Work out the finished part from the listing and answer in its coordinate system (mm). Give positions to 0.01 mm unless a question says otherwise; leave off trailing zeros. Write each loop counter-clockwise with the first axis right and the second up, starting at its lowest first coordinate (ties: lowest second). Pieces come first, ordered by that corner, then holes. Notation, with made-up numbers: (5.25, -28.5) - (24.25, -28.5) arc R12 cw to (24.25, -7.5) - close; hole circle Ø8 at (64.25, -7). An arc over 180 degrees is marked (long way). Write each question's results on one line, items separated by ' | '. Start each with the question number.
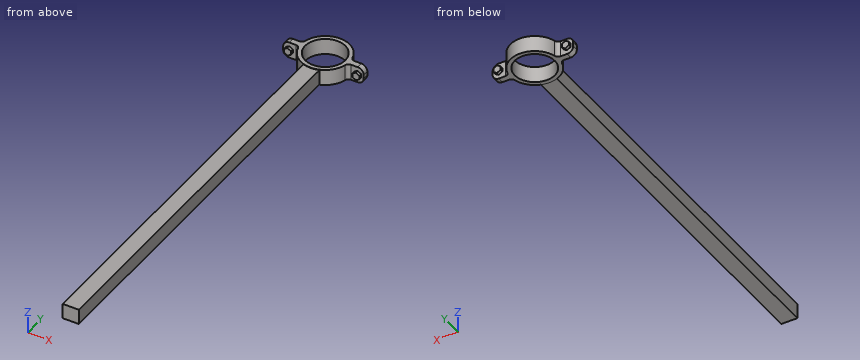
Autodesk Inventor part; units mm, degrees
ref_plane "Arbeitsebene1" through (0, -52.25, 0) normal (0, 1, 0) x (-1, 0, 0)
ref_plane "YZ Plane" through (0, 0, 0) normal (1, 0, 0) x (0, 1, 0)
ref_plane "XY Plane" through (0, 0, 0) normal (0, 0, 1) x (1, 0, 0)
sketch "Skizze1" plane through (0, 0, 0) normal (0, 0, 1) x (1, 0, 0)
  circle A0 centre (0, 0) radius 50
  line L0 (100, 7.5) -> (100, -7.5)
  line L1 (-100, -7.5) -> (-100, 7.5)
  line L2 (-100, 7.5) -> (-68.374, 7.5)
  line L3 (68.374, 7.5) -> (100, 7.5)
  line L4 (100, -7.5) -> (68.374, -7.5)
  line L5 (-68.374, -7.5) -> (-100, -7.5)
  arc A1 (-58.6863, -15.0205) -> (58.6863, -15.0205) centre (0, 0) ccw
  arc A2 (58.6863, 15.0205) -> (-58.6863, 15.0205) centre (0, 0) ccw
  arc A3 (-68.374, 7.5) -> (-58.6863, 15.0205) centre (-68.374, 17.5) ccw
  arc A4 (-58.6863, -15.0205) -> (-68.374, -7.5) centre (-68.374, -17.5) ccw
  arc A5 (58.6863, 15.0205) -> (68.374, 7.5) centre (68.374, 17.5) ccw
  arc A6 (68.374, -7.5) -> (58.6863, -15.0205) centre (68.374, -17.5) ccw
  point P0 (-60.1119, 7.5)
  point P1 (60.1119, 7.5)
  point P2 (60.1119, -7.5)
  point P3 (-60.1119, -7.5)
  point P4 (-84.187, 7.5)
  point P5 (84.187, 7.5)
  point P6 (84.187, -7.5)
  point P7 (-84.187, -7.5)
  dimension "d1" = 100
  dimension "d4" = 100
  dimension "d5" = 100
  dimension "d6" = 10
  dimension "d7" = 7.5
  dimension "d8" = 7.5
extrude "Extrusion1" add sketch "Skizze1" along normal blind 40
fillet "Rundung1" radius 15 4 edges at (100, 0, 40) (100, 0, 0) (-100, 0, 40) (-100, 0, 0)
sketch "Skizze3" plane through (0, 0, 0) normal (0, 1, 0) x (-1, 0, 0)
  circle A0 centre (-85, 20) radius 10 construction
  line L0 (-85, 10) -> (-93.7649, 15.1858)
  line L1 (-93.7649, 24.8142) -> (-85, 30)
  line L2 (-85, 30) -> (-76.2351, 24.8142)
  line L3 (-76.2351, 24.8142) -> (-76.2351, 15.1858)
  line L4 (-85, 10) -> (-76.2351, 15.1858)
  line L5 (-93.7649, 24.8142) -> (-93.7649, 15.1858)
  arc A1 (-100, 15) -> (-85, 0) centre (-85, 15) ccw
  line L6 (-85, 0) -> (-68.374, 0)
  line L7 (-68.374, 0) -> (-68.374, 40)
  line L8 (-85, 40) -> (-68.374, 40)
  arc A2 (-85, 40) -> (-100, 25) centre (-85, 25) ccw
  line L9 (-100, 15) -> (-100, 25)
  arc A3 (85, 0) -> (100, 15) centre (85, 15) ccw
  line L10 (100, 15) -> (100, 25)
  arc A4 (100, 25) -> (85, 40) centre (85, 25) ccw
  line L11 (68.374, 40) -> (85, 40)
  line L12 (68.374, 0) -> (68.374, 40)
  line L13 (68.374, 0) -> (85, 0)
  line L14 (-85, 15) -> (-85, 25) construction
  line L15 (85, 15) -> (85, 25) construction
  circle A5 centre (85, 20) radius 10 construction
  line L16 (85, 10) -> (76.2351, 15.1858)
  line L17 (76.2351, 24.8142) -> (85, 30)
  line L18 (85, 30) -> (93.7649, 24.8142)
  line L19 (93.7649, 24.8142) -> (93.7649, 15.1858)
  line L20 (85, 10) -> (93.7649, 15.1858)
  line L21 (76.2351, 24.8142) -> (76.2351, 15.1858)
  line L22 (85, 15) -> (85, 25) construction
  point P0 (0, 0)
  point P1 (85, 20)
  dimension "d12" = 20
  dimension "d13" = 20
extrude "Extrusion2" add sketch "Skizze3" along normal mid plane 30 contours L0 L5 L1 L2 L3 L4 | L16 L21 L17 L18 L19 L20
ref_plane "Arbeitsebene1" through (0, -52.25, 0) normal (0, 1, 0) x (-1, 0, 0)
sketch "Skizze4" plane through (0, -52.25, 0) normal (0, 1, 0) x (-1, 0, 0)
  line L0 (20, 39) -> (-20, 39)
  line L1 (-20, 39) -> (-20, 1)
  line L2 (-20, 1) -> (20, 1)
  line L3 (20, 1) -> (20, 39)
  point P0 (0, 0)
  dimension "d22" = 1
  dimension "d23" = 38
  dimension "d24" = 20
  dimension "d25" = 20
extrude "Extrusion3" add sketch "Skizze4" against normal blind 1000
properties part number "DN80-Rohrschelle-Staender"
Q1. A cutting plane is placed at A-A, the plane x = 0. Write down the section's boundary in (y, z).
Q2. Given pin 1 (8 mm diameter, centred on y = 12, z = 18.5, fed in from +X); pin 2 (1 mm diameter, centred on y = -658.5, z = 26.5, fed in from -X); pin 3 (9.5 mm diameter, centred on x = 78, z = 19, fed in from +Y), each flat-ended and moving along its own axis, determine where each tip first touches the part or whether it passes through.
Q3. Consider L1, parallel to Y at x = 1.5, z = 8; L2, parallel to X at y = -915, z = 10; L3, parallel to Y at x = -39, z = 37. Determine where each line is inside the solid, lowest interval first.
Q4. A cutting plane is placed at B-B, the plane y = -856.5. Write down the section's boundary in (x, z), and give its area (3 significant figures).
Result:
1) outline: (-1052.25, 1) - (-60.58, 1) - (-60.58, 0) - (-50, 0) - (-50, 40) - (-60.58, 40) - (-60.58, 39) - (-1052.25, 39) - close; (50, 0) - (60.58, 0) - (60.58, 40) - (50, 40) - close
2) pin 1: stops at x = 93.76 | pin 2: stops at x = -20 | pin 3: stops at y = 15
3) L1: y = -1052.25 to -49.98, 49.98 to 60.56 | L2: x = -20 to 20 | L3: y = -46.35 to -31.29, 31.29 to 46.35
4) outline: (-20, 1) - (20, 1) - (20, 39) - (-20, 39) - close | area: 1,520 mm2
